Verification items for the finished model (mm, model axes). Round coordinates to 2 decimals unless told otherwise and drop trailing zeros. Order: outer loops, then holes, each group sorted by start corner. A loop starts at its lowest first (then second) coordinate and runs counter-clockwise, first axis right, second up. Notation, with made-up numbers: M 81.25,11.25 L 110.25,11.25 A17 ccw 110.25,15.25 Z; hole C 39.25,-9 d5. An arc over 180 degrees is marked long. Use one line per item in the form item = value. Start each with the question number.
Item 1: Cross-section at A-A on z = 76. Enter the section's corners in (x, y), then the cut area to 3 significant figures.
Item 2: Release check for a two-part mould opening along X. For faces 1 (the cylindrical face through (255.36, 400.52, 49.3)), 2 (the flat face through (-354, -318, 0)), 3 (the cylindrical face through (221.95, -426.73, 50.7)) record: +X half, -X half, draft (parallel to the pull), parting line (faces both ways), or undercut.
Item 3: Thickness scan on probe 1 along Y at (x, z) = (0, 71); probe 2 along Y at (x, z) = (-312, 76.5); probe 3 along X at (y, z) = (279, 128). Record the ranges inside material, lowest first. Write a range as [from, to].
Item 4: Go/stop test with flat-tipped pins: pin 1 Ø5 at (x, z) = (257.5, 108) entering from +Y; pin 2 Ø1 at (x, z) = (298.5, 163.5) entering from -Y; pin 3 Ø4 at (y, z) = (299.5, 172) entering from +X. Record where each tip stops, or that it passes through.
from build123d import *


with BuildPart() as f1:
    # F0 (on Front) → F1 (revolve)
    with BuildSketch(Plane.XZ):
        with BuildLine():
            ThreePointArc((419.117647, 189.742037), (459.887469, 152.859414), (475, 100))
            Line((475, 100), (475, 0))
            Line((475, 0), (481, 0))
            Line((481, 0), (481, 100))
            ThreePointArc((481, 100), (464.980717, 156.030979), (421.764706, 195.126559))
            ThreePointArc((421.764706, 195.126559), (216.507755, 268.353462), (0, 293.192685))
            Line((0, 293.192685), (0, 287.192685))
            ThreePointArc((0, 287.192685), (215.14892, 262.509356), (419.117647, 189.742037))
        make_face()
    revolve(axis=Axis((0, 0, 568.160451), (0, 0, 1)))


solid = f1.part
Output values:
q1.outline = C 0,0 d962; hole C 0,0 d950
q1.area = 18,000 mm2
q2.face_1 = undercut
q2.face_2 = draft
q2.face_3 = parting line
q3.probe_1 = [-481, -475], [475, 481]
q3.probe_2 = [-366.08, -358.16], [358.16, 366.08]
q3.probe_3 = [-387.19, -379.47], [379.47, 387.19]
q4.pin_1 = 407.5
q4.pin_2 = -350.48
q4.pin_3 = 342.57
